Input: part model. Units: mm. Frame: model coordinates. Face numbers are marked on the shaded views. A direction names the side the tool comes from. Give positions to 0.01 mm unless a question says otherwise; leave off trailing zeros. Write each loop counter-clockwise with the first axis right and the second up, starting at its lowest first coordinate (ties: lowest second). Pieces come first, ordered by that corner, then holes. Notation, with made-up numbers: (60.5, 4.5) - (111.5, 4.5) arc R28 cw to (111.5, 29.5) - close; hole circle Ø3 at (89, 75). An arc over 180 degrees is marked (long way). Answer as a JSON object with one key per item and string values. Group by question number.
from build123d import *

# Parameters (mm, degrees)
PATTERN_CIRCULAR_2_COUNT = 4
CHAMFER_1_SIZE           = 2


with BuildPart() as part:
    # Эскиз1 → Повернуть1 (revolve)
    with BuildSketch(Plane.XY, mode=Mode.PRIVATE) as revolve_1_sk:
        Polygon((0, 7), (0, 15), (12, 15), (12, 4.5), (8, 4.5), (8, 7), align=None)
    revolve(revolve_1_sk.sketch.rotate(Axis((0, 0, 0), (1, 0, 0)), 90), axis=Axis((0, 0, 0), (1, 0, 0)))

    # Эскиз3 → Отверстия под штифты Ø4.0 мм1 (revolve, cut)
    with BuildSketch(Plane(origin=(12, 10, 0), x_dir=(0, 0, -1), z_dir=(0, 1, 0))):
        Polygon((0, 0), (0, 6.201721238), (2, 5), (2, 0.025), (2.025, 0), align=None)
    hole_wizard_4_0_1 = revolve(axis=Axis((18.35, 10, 0), (-1, 0, 0)), mode=Mode.SUBTRACT)

    # Круговой массив2: Отверстия под штифты Ø4.0 мм1 ×4 about axis
    pattern_circular_2_axis = Axis((0, 0, 0), (1, 0, 0))
    for i in range(1, PATTERN_CIRCULAR_2_COUNT):
        add(hole_wizard_4_0_1.rotate(pattern_circular_2_axis, i * 360 / PATTERN_CIRCULAR_2_COUNT), mode=Mode.SUBTRACT)

    # Фаска1
    chamfer_1_edges = [part.edges().sort_by_distance(p)[0] for p in [
        (12, 0, -15),
        (0, 0, -15),
    ]]
    chamfer(chamfer_1_edges, length=CHAMFER_1_SIZE)


solid = part.part
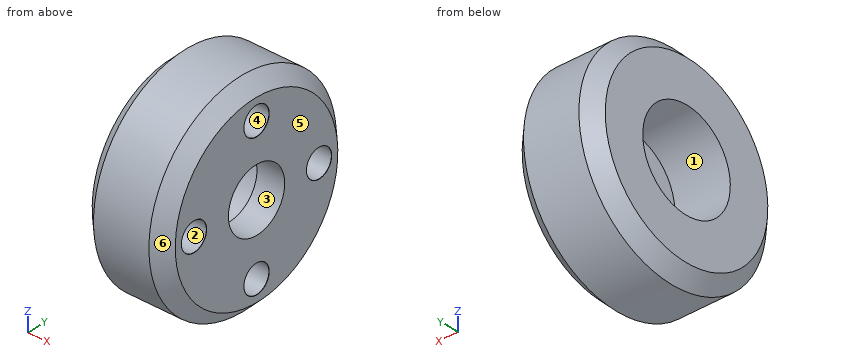
1) Line query: line 1 along Y through (x, z) = (3, 0); line 2 along Y through (x, z) = (10.75, 0); line 3 along Z through (x, y) = (6.25, -5). Output: solid intervals per line, ascending. Write a range as from..to.
2) Pin query (flat end, axial travel): P1, Ø3, axis at x = 1.5, z = -6.5, coming from the +Y side; P2, Ø4, axis at x = 3, y = -5.5, coming from the -Z side; P3, Ø3.5, axis at y = 10, z = 0, coming from the +X side. Return the tip coordinate at first contact, or that it passes through.
3) Cut plane C-C on x = 11. Return the cut outline in (y, z).
4) Reachability of the marked faces 1, 2 and 3 from +Z, -Z, +X, -X, +Y, -Y: full face, straight path, thin tool, end or side. Return the list, or none.
5) Mould query, pull axis Z, two halves, no side actions, for the marked faces 4, 5 and 6. Classes: +Z half, -Z half, draft (parallel to the pull), parting line (faces both ways), or undercut.
6) Cut plane B-B on x = 3.75. Return the cut outline in (y, z).
7) Cut plane A-A on x = 8.75. Return the cut outline in (y, z).
Filled in:
{
 "1": {"line 1": "y = -15..-7, 7..15", "line 2": "y = -14.25..-12, -8..-4.5, 4.5..8, 12..14.25", "line 3": "z = -14.14..-4.9, 4.9..14.14"},
 "2": {"P1": "stops at y = 14.11", "P2": "stops at z = -14.59", "P3": "stops at x = 6.85"},
 "3": {"outline": "circle Ø28 at (0, 0); hole circle Ø4 at (-10, 0); hole circle Ø9 at (0, 0); hole circle Ø4 at (0, -10); hole circle Ø4 at (0, 10); hole circle Ø4 at (10, 0)"},
 "4": {"face 1": "-X", "face 2": "+X", "face 3": "+X, -X"},
 "5": {"face 4": "undercut", "face 5": "draft", "face 6": "parting line"},
 "6": {"outline": "circle Ø30 at (0, 0); hole circle Ø14 at (0, 0)"},
 "7": {"outline": "circle Ø30 at (0, 0); hole circle Ø4 at (-10, 0); hole circle Ø9 at (0, 0); hole circle Ø4 at (0, -10); hole circle Ø4 at (0, 10); hole circle Ø4 at (10, 0)"}
}
